```python
from build123d import *

# Parameters (mm, degrees)
ESQUISSE1_R      = 2.15
EXTRUSION1_DEPTH = 445.3


with BuildPart() as part:
    # Esquisse1 → Extrusion1 (new body)
    with BuildSketch(Plane(origin=(0, 0, 0), x_dir=(-1, 0, 0), z_dir=(0, 0, -1))):
        with BuildLine():
            Line((-38, 0), (-33.3, 0))
            ThreePointArc((-33.3, 0), (-32.734314575, 0.234314575), (-32.5, 0.8))
            Line((-32.5, 0.8), (-32.5, 1.5))
            ThreePointArc((-32.5, 1.5), (-32.587867966, 1.712132034), (-32.8, 1.8))
            Line((-32.8, 1.8), (-34.918424061, 1.8))
            ThreePointArc((-34.918424061, 1.8), (-35.686700051, 2.313345604), (-35.506437047, 3.219588924))
            Line((-35.506437047, 3.219588924), (-33.254705627, 5.471320344))
            ThreePointArc((-33.254705627, 5.471320344), (-32.281435581, 6.121638598), (-31.133385284, 6.35))
            Line((-31.133385284, 6.35), (-28.866614716, 6.35))
            ThreePointArc((-28.866614716, 6.35), (-27.718564419, 6.121638598), (-26.745294373, 5.471320344))
            Line((-26.745294373, 5.471320344), (-24.493562953, 3.219588924))
            ThreePointArc((-24.493562953, 3.219588924), (-24.313299949, 2.313345604), (-25.081575939, 1.8))
            Line((-25.081575939, 1.8), (-27.2, 1.8))
            ThreePointArc((-27.2, 1.8), (-27.412132034, 1.712132034), (-27.5, 1.5))
            Line((-27.5, 1.5), (-27.5, 0.8))
            ThreePointArc((-27.5, 0.8), (-27.265685425, 0.234314575), (-26.7, 0))
            Line((-26.7, 0), (-13.3, 0))
            ThreePointArc((-13.3, 0), (-12.734314575, 0.234314575), (-12.5, 0.8))
            Line((-12.5, 0.8), (-12.5, 1.5))
            ThreePointArc((-12.5, 1.5), (-12.587867966, 1.712132034), (-12.8, 1.8))
            Line((-12.8, 1.8), (-14.918424061, 1.8))
            ThreePointArc((-14.918424061, 1.8), (-15.686700051, 2.313345604), (-15.506437047, 3.219588924))
            Line((-15.506437047, 3.219588924), (-13.254705627, 5.471320344))
            ThreePointArc((-13.254705627, 5.471320344), (-12.281435581, 6.121638598), (-11.133385284, 6.35))
            Line((-11.133385284, 6.35), (-8.866614716, 6.35))
            ThreePointArc((-8.866614716, 6.35), (-7.718564419, 6.121638598), (-6.745294373, 5.471320344))
            Line((-6.745294373, 5.471320344), (-4.493562953, 3.219588924))
            ThreePointArc((-4.493562953, 3.219588924), (-4.313299949, 2.313345604), (-5.081575939, 1.8))
            Line((-5.081575939, 1.8), (-7.2, 1.8))
            ThreePointArc((-7.2, 1.8), (-7.412132034, 1.712132034), (-7.5, 1.5))
            Line((-7.5, 1.5), (-7.5, 0.8))
            ThreePointArc((-7.5, 0.8), (-7.265685425, 0.234314575), (-6.7, 0))
            Line((-6.7, 0), (-2, 0))
            ThreePointArc((-2, 0), (-0.585786438, 0.585786438), (0, 2))
            Line((0, 2), (0, 6.7))
            ThreePointArc((0, 6.7), (-0.234314575, 7.265685425), (-0.8, 7.5))
            Line((-0.8, 7.5), (-1.5, 7.5))
            ThreePointArc((-1.5, 7.5), (-1.712132034, 7.412132034), (-1.8, 7.2))
            Line((-1.8, 7.2), (-1.8, 5.081575939))
            ThreePointArc((-1.8, 5.081575939), (-2.313345604, 4.313299949), (-3.219588924, 4.493562953))
            Line((-3.219588924, 4.493562953), (-5.471320344, 6.745294373))
            ThreePointArc((-5.471320344, 6.745294373), (-6.121638598, 7.718564419), (-6.35, 8.866614716))
            Line((-6.35, 8.866614716), (-6.35, 11.133385284))
            ThreePointArc((-6.35, 11.133385284), (-6.121638598, 12.281435581), (-5.471320344, 13.254705627))
            Line((-5.471320344, 13.254705627), (-3.219588924, 15.506437047))
            ThreePointArc((-3.219588924, 15.506437047), (-2.313345604, 15.686700051), (-1.8, 14.918424061))
            Line((-1.8, 14.918424061), (-1.8, 12.8))
            ThreePointArc((-1.8, 12.8), (-1.712132034, 12.587867966), (-1.5, 12.5))
            Line((-1.5, 12.5), (-0.8, 12.5))
            ThreePointArc((-0.8, 12.5), (-0.234314575, 12.734314575), (0, 13.3))
            Line((0, 13.3), (0, 18))
            ThreePointArc((0, 18), (-0.585786438, 19.414213562), (-2, 20))
            Line((-2, 20), (-6.7, 20))
            ThreePointArc((-6.7, 20), (-7.265685425, 19.765685425), (-7.5, 19.2))
            Line((-7.5, 19.2), (-7.5, 18.5))
            ThreePointArc((-7.5, 18.5), (-7.412132034, 18.287867966), (-7.2, 18.2))
            Line((-7.2, 18.2), (-5.081575939, 18.2))
            ThreePointArc((-5.081575939, 18.2), (-4.313299949, 17.686654396), (-4.493562953, 16.780411076))
            Line((-4.493562953, 16.780411076), (-6.745294373, 14.528679656))
            ThreePointArc((-6.745294373, 14.528679656), (-7.718564419, 13.878361402), (-8.866614716, 13.65))
            Line((-8.866614716, 13.65), (-11.133385284, 13.65))
            ThreePointArc((-11.133385284, 13.65), (-12.281435581, 13.878361402), (-13.254705627, 14.528679656))
            Line((-13.254705627, 14.528679656), (-15.506437047, 16.780411076))
            ThreePointArc((-15.506437047, 16.780411076), (-15.686700051, 17.686654396), (-14.918424061, 18.2))
            Line((-14.918424061, 18.2), (-12.8, 18.2))
            ThreePointArc((-12.8, 18.2), (-12.587867966, 18.287867966), (-12.5, 18.5))
            Line((-12.5, 18.5), (-12.5, 19.2))
            ThreePointArc((-12.5, 19.2), (-12.734314575, 19.765685425), (-13.3, 20))
            Line((-13.3, 20), (-26.7, 20))
            ThreePointArc((-26.7, 20), (-27.265685425, 19.765685425), (-27.5, 19.2))
            Line((-27.5, 19.2), (-27.5, 18.5))
            ThreePointArc((-27.5, 18.5), (-27.412132034, 18.287867966), (-27.2, 18.2))
            Line((-27.2, 18.2), (-25.081575939, 18.2))
            ThreePointArc((-25.081575939, 18.2), (-24.313299949, 17.686654396), (-24.493562953, 16.780411076))
            Line((-24.493562953, 16.780411076), (-26.745294373, 14.528679656))
            ThreePointArc((-26.745294373, 14.528679656), (-27.718564419, 13.878361402), (-28.866614716, 13.65))
            Line((-28.866614716, 13.65), (-31.133385284, 13.65))
            ThreePointArc((-31.133385284, 13.65), (-32.281435581, 13.878361402), (-33.254705627, 14.528679656))
            Line((-33.254705627, 14.528679656), (-35.506437047, 16.780411076))
            ThreePointArc((-35.506437047, 16.780411076), (-35.686700051, 17.686654396), (-34.918424061, 18.2))
            Line((-34.918424061, 18.2), (-32.8, 18.2))
            ThreePointArc((-32.8, 18.2), (-32.587867966, 18.287867966), (-32.5, 18.5))
            Line((-32.5, 18.5), (-32.5, 19.2))
            ThreePointArc((-32.5, 19.2), (-32.734314575, 19.765685425), (-33.3, 20))
            Line((-33.3, 20), (-38, 20))
            ThreePointArc((-38, 20), (-39.414213562, 19.414213562), (-40, 18))
            Line((-40, 18), (-40, 13.3))
            ThreePointArc((-40, 13.3), (-39.765685425, 12.734314575), (-39.2, 12.5))
            Line((-39.2, 12.5), (-38.5, 12.5))
            ThreePointArc((-38.5, 12.5), (-38.287867966, 12.587867966), (-38.2, 12.8))
            Line((-38.2, 12.8), (-38.2, 14.918424061))
            ThreePointArc((-38.2, 14.918424061), (-37.686654396, 15.686700051), (-36.780411076, 15.506437047))
            Line((-36.780411076, 15.506437047), (-34.528679656, 13.254705627))
            ThreePointArc((-34.528679656, 13.254705627), (-33.878361402, 12.281435581), (-33.65, 11.133385284))
            Line((-33.65, 11.133385284), (-33.65, 8.866614716))
            ThreePointArc((-33.65, 8.866614716), (-33.878361402, 7.718564419), (-34.528679656, 6.745294373))
            Line((-34.528679656, 6.745294373), (-36.780411076, 4.493562953))
            ThreePointArc((-36.780411076, 4.493562953), (-37.686654396, 4.313299949), (-38.2, 5.081575939))
            Line((-38.2, 5.081575939), (-38.2, 7.2))
            ThreePointArc((-38.2, 7.2), (-38.287867966, 7.412132034), (-38.5, 7.5))
            Line((-38.5, 7.5), (-39.2, 7.5))
            ThreePointArc((-39.2, 7.5), (-39.765685425, 7.265685425), (-40, 6.7))
            Line((-40, 6.7), (-40, 2))
            ThreePointArc((-40, 2), (-39.414213562, 0.585786438), (-38, 0))
        make_face()
        with Locations(Location((-10, 10, 0), (0, 0, 180))):
            Circle(ESQUISSE1_R, mode=Mode.SUBTRACT)
        with Locations(Location((-30, 10, 0), (0, 0, 180))):
            Circle(ESQUISSE1_R, mode=Mode.SUBTRACT)
        with BuildLine():
            Line((-13.650001154, 11.134569154), (-13.650001154, 8.865431094))
            ThreePointArc((-13.650001154, 8.865431094), (-13.878362476, 7.717381202), (-14.5286805, 6.7441115))
            Line((-14.5286805, 6.7441115), (-18.585786, 2.687006))
            ThreePointArc((-18.585786, 2.687006), (-19.999999562, 2.101219562), (-21.414213125, 2.687006))
            Line((-21.414213125, 2.687006), (-25.471320125, 6.744113))
            ThreePointArc((-25.471320125, 6.744113), (-26.121638379, 7.717383046), (-26.349999781, 8.865433344))
            Line((-26.349999781, 8.865433344), (-26.349999781, 11.134567344))
            ThreePointArc((-26.349999781, 11.134567344), (-26.121638308, 12.282617811), (-25.471319863, 13.255887949))
            Line((-25.471319863, 13.255887949), (-21.41421295, 17.312993861))
            ThreePointArc((-21.41421295, 17.312993861), (-19.999999562, 17.898780125), (-18.585786174, 17.312993861))
            Line((-18.585786174, 17.312993861), (-14.528681072, 13.255889759))
            ThreePointArc((-14.528681072, 13.255889759), (-13.878362627, 12.282619622), (-13.650001154, 11.134569154))
        make_face(mode=Mode.SUBTRACT)
    extrude(amount=-EXTRUSION1_DEPTH)


solid = part.part
```
Can you work these out from the model? Positions are in its coordinate system, mm. Round coordinates to 2 decimals unless told otherwise and drop trailing zeros. One line per item, written item: value. Start each with the question number.
1. If we section it at A-A, the plane z = 224.5: Give the number of separate pieces and of enclosed holes in the cut face, then the cut area to 3 significant figures.
2. If I drill on probe 1 along X at (y, z) = (10, 137); probe 2 along Y at (x, z) = (10, 307.5); probe 3 along Y at (x, z) = (35, 55.5), over which ranges is the centre line in solid material (lowest first)?
3. For pin 1 (2.5 mm diameter, centred on y = 10, z = 249, fed in from +X); pin 2 (2.5 mm diameter, centred on y = 10, z = 206.5, fed in from -X); pin 3 (0.6 mm diameter, centred on x = 1, z = 254.5, fed in from -Y), each with a flat end and sliding along its axis, tell me the tip position at first contact or that it passes through.
Calculated:
1. separate pieces: 1
1. enclosed holes: 3
1. area: 332 mm²
2. probe 1: x = 6.35 to 7.85, 12.15 to 13.65, 26.35 to 27.85, 32.15 to 33.65
2. probe 2: y = 6.35 to 7.85, 12.15 to 13.65
2. probe 3: y = 0 to 1.8, 3.73 to 6.27, 13.73 to 16.27, 18.2 to 20
3. pin 1: stops at x = 33.65
3. pin 2: stops at x = 6.35
3. pin 3: stops at y = 0.13
